For this review, take the finished solid that the model builds, in its own axes (mm). A direction names the side the tool comes from. Coordinates: 2 decimals unless noted, no trailing zeros. Write each loop counter-clockwise with the first axis right and the second up, starting at its lowest first coordinate (ties: lowest second). Pieces come first, ordered by that corner, then holes. Notation, with made-up numbers: M -10,71 L 5,71 A26 cw 5,92 Z; hole C -18,17.5 d3. An arc over 180 degrees is marked long. One line per question, with ' | ' between items.
from build123d import *

# Parameters (mm, degrees)
SKETCH1_W           = 50
SKETCH1_H           = 75
BOSS_EXTRUDE1_DEPTH = 20
SHELL1_T            = -2
FILLET1_R           = 2
SKETCH2_R           = 12.5
BOSS_EXTRUDE2_DEPTH = 1
FILLET2_R           = 2
CUT_EXTRUDE1_DEPTH  = 5
SKETCH4_R           = 2.084715902
SKETCH4_R_2         = 2.544136108
SKETCH4_R_3         = 2.861924979
SKETCH4_R_4         = 2.414925707
BOSS_EXTRUDE3_DEPTH = 7
CHAMFER1_SIZE       = 2
CUT_EXTRUDE2_DEPTH  = 4
SKETCH7_W           = 2
SKETCH7_H           = 1.627577662
BOSS_EXTRUDE4_DEPTH = 3
SKETCH8_W           = 2
SKETCH8_H           = 1.808898565
BOSS_EXTRUDE5_DEPTH = 3
SKETCH9_R           = 0.5
CUT_EXTRUDE3_DEPTH  = 2
CUT_EXTRUDE4_START  = -2
CUT_EXTRUDE4_DEPTH  = 2
SKETCH12_W          = 8.5
SKETCH12_H          = 4
CUT_EXTRUDE5_DEPTH  = 3
SKETCH14_W          = 10
SKETCH14_H          = 2.18902829
CUT_EXTRUDE7_DEPTH  = 3
SKETCH15_W          = 10
SKETCH15_H          = 2.825004844
CUT_EXTRUDE8_DEPTH  = 0.5
CUT_EXTRUDE9_DEPTH  = 3


with BuildPart() as part:
    # Sketch1 → Boss-Extrude1 (new body)
    with BuildSketch(Plane(origin=(0, 0, 0), x_dir=(1, 0, 0), z_dir=(0, 1, 0))):
        with Locations((25, 37.5)):
            Rectangle(SKETCH1_W, SKETCH1_H)
    extrude(amount=BOSS_EXTRUDE1_DEPTH)

    # Shell1
    shell1_openings = [part.faces().sort_by_distance(p)[0] for p in [
        (25, 20, -37.5),
    ]]
    offset(amount=SHELL1_T, openings=shell1_openings, kind=Kind.INTERSECTION)

    # Fillet1
    fillet1_edges = [part.edges().sort_by_distance(p)[0] for p in [
        (0, 10, -75),
        (50, 10, -75),
        (50, 10, 0),
        (0, 10, 0),
    ]]
    fillet(fillet1_edges, radius=FILLET1_R)

    # Sketch2 → Boss-Extrude2 (add)
    with BuildSketch(Plane.XZ):
        with Locations(Location((25, -37.5, 0), (0, 0, 270))):
            Circle(SKETCH2_R)
    extrude(amount=BOSS_EXTRUDE2_DEPTH)

    # Fillet2
    # the kernel refuses this fillet: 2 mm, written as the material it takes off along each edge
    with BuildSketch(Plane(origin=(25, -1, -37.5), x_dir=(0, 0, -1), z_dir=(-1, 0, 0))) as fillet2_piece_1:
        with BuildLine():
            CenterArc((10.767949192, -2), FILLET2_R, 30, 60)
            Line((10.767949192, 0), (10.767949192, 0.04))
            Line((10.767949192, 0.04), (12.5, 0.04))
            Line((12.5, 0.04), (12.54, 0))
            ThreePointArc((12.54, 0), (12.54, -0.5), (12.534641016, -0.98))
            Line((12.534641016, -0.98), (12.5, -1))
        make_face()
    revolve(axis=Axis((25, -1, -37.5), (0, -1, 0)), mode=Mode.SUBTRACT)

    # Sketch3 → Cut-Extrude1 (cut)
    with BuildSketch(Plane.XZ.offset(1)):
        Polygon((33, -40), (33, -37.5), (33, -35), (25.072423756, -35), (25.072423756, -37.5), (25.072423756, -40), align=None)
    extrude(amount=-CUT_EXTRUDE1_DEPTH, mode=Mode.SUBTRACT)

    # Sketch4 → Boss-Extrude3 (add)
    with BuildSketch(Plane(origin=(0, 2, 0), x_dir=(1, 0, 0), z_dir=(0, 1, 0))):
        with Locations(Location((7, 65.5, 0), (0, 0, 90))):
            Circle(SKETCH4_R)
        with Locations(Location((43, 65.5, 0), (0, 0, 90))):
            Circle(SKETCH4_R_2)
        with Locations(Location((43, 9.5, 0), (0, 0, 90))):
            Circle(SKETCH4_R_3)
        with Locations(Location((7, 9.5, 0), (0, 0, 90))):
            Circle(SKETCH4_R_4)
    extrude(amount=BOSS_EXTRUDE3_DEPTH)

    # Chamfer1
    chamfer1_edges = [part.edges().sort_by_distance(p)[0] for p in [
        (33, 2, -37.5),
        (29.036211878, 2, -40),
        (29.036211878, 2, -35),
        (25.072423756, 2, -37.5),
    ]]
    chamfer(chamfer1_edges, length=CHAMFER1_SIZE)

    # Sketch5 → Cut-Extrude2 (cut)
    with BuildSketch(Plane.ZY):
        Polygon((-37.5, 0), (-27.5, 0), (-27.5, 5), (-47.5, 5), (-47.5, 0), align=None)
    cut_extrude2 = extrude(amount=-CUT_EXTRUDE2_DEPTH, mode=Mode.SUBTRACT)

    # Sketch7 → Boss-Extrude4 (add)
    with BuildSketch(Plane(origin=(0, 2, 0), x_dir=(1, 0, 0), z_dir=(0, 1, 0))):
        with Locations((3, 48.313788831)):
            Rectangle(SKETCH7_W, SKETCH7_H)
    boss_extrude4 = extrude(amount=BOSS_EXTRUDE4_DEPTH)

    # Sketch8 → Boss-Extrude5 (add)
    with BuildSketch(Plane(origin=(0, 2, 0), x_dir=(1, 0, 0), z_dir=(0, 1, 0))):
        with Locations((3, 26.595550718)):
            Rectangle(SKETCH8_W, SKETCH8_H)
    boss_extrude5 = extrude(amount=BOSS_EXTRUDE5_DEPTH)

    # Sketch9 → Cut-Extrude3 (cut)
    with BuildSketch(Plane.XY.offset(-47.5)):
        with Locations((2, 4)):
            Circle(SKETCH9_R)
    cut_extrude3 = extrude(amount=-CUT_EXTRUDE3_DEPTH, mode=Mode.SUBTRACT)

    # Sketch10 → Cut-Extrude4 (cut)
    with BuildSketch(Plane(origin=(0, 0, -27.5), x_dir=(-1, 0, 0), z_dir=(0, 0, -1)).offset(CUT_EXTRUDE4_START)):
        with BuildLine():
            ThreePointArc((-1.5, 4), (-1.646446609, 4.353553391), (-2, 4.5))
            Line((-2, 4.5), (-2, 3.5))
            ThreePointArc((-2, 3.5), (-1.646446609, 3.646446609), (-1.5, 4))
        make_face()
        with BuildLine():
            Line((-2, 3.5), (-2, 4.5))
            ThreePointArc((-2, 4.5), (-2.5, 4), (-2, 3.5))
        make_face()
    cut_extrude4 = extrude(amount=CUT_EXTRUDE4_DEPTH, mode=Mode.SUBTRACT)

    # Mirror1: Cut-Extrude2, Boss-Extrude4, Boss-Extrude5, Cut-Extrude3, Cut-Extrude4 across plane
    add(cut_extrude2.mirror(Plane(origin=(25, 0, 0), x_dir=(0, 0, 1), z_dir=(1, 0, 0))), mode=Mode.SUBTRACT)
    add(boss_extrude4.mirror(Plane(origin=(25, 0, 0), x_dir=(0, 0, 1), z_dir=(1, 0, 0))))
    add(boss_extrude5.mirror(Plane(origin=(25, 0, 0), x_dir=(0, 0, 1), z_dir=(1, 0, 0))))
    add(cut_extrude3.mirror(Plane(origin=(25, 0, 0), x_dir=(0, 0, 1), z_dir=(1, 0, 0))), mode=Mode.SUBTRACT)
    add(cut_extrude4.mirror(Plane(origin=(25, 0, 0), x_dir=(0, 0, 1), z_dir=(1, 0, 0))), mode=Mode.SUBTRACT)

    # Sketch12 → Cut-Extrude5 (cut)
    with BuildSketch(Plane.ZY):
        with Locations((-53.834118064, 7.735405472)):
            Rectangle(SKETCH12_W, SKETCH12_H)
    extrude(amount=-CUT_EXTRUDE5_DEPTH, mode=Mode.SUBTRACT)

    # Sketch14 → Cut-Extrude7 (cut)
    with BuildSketch(Plane(origin=(0, 0, -2), x_dir=(-1, 0, 0), z_dir=(0, 0, -1))):
        with Locations((-25, 15.905485855)):
            Rectangle(SKETCH14_W, SKETCH14_H)
    cut_extrude7 = extrude(amount=-CUT_EXTRUDE7_DEPTH, mode=Mode.SUBTRACT)

    # Sketch15 → Cut-Extrude8 (cut)
    with BuildSketch(Plane(origin=(2, 0, 0), x_dir=(0, 0, -1), z_dir=(1, 0, 0))):
        with Locations((37.5, 15.587497578)):
            Rectangle(SKETCH15_W, SKETCH15_H)
    cut_extrude8 = extrude(amount=-CUT_EXTRUDE8_DEPTH, mode=Mode.SUBTRACT)

    # Mirror2: Cut-Extrude7 across plane
    add(cut_extrude7.mirror(Plane.XY.offset(-37.5)), mode=Mode.SUBTRACT)

    # Mirror3: Cut-Extrude8 across plane
    add(cut_extrude8.mirror(Plane(origin=(25, 0, 0), x_dir=(0, 0, 1), z_dir=(1, 0, 0))), mode=Mode.SUBTRACT)

    # Sketch16 → Cut-Extrude9 (cut)
    with BuildSketch(Plane(origin=(0, 0, -75), x_dir=(-1, 0, 0), z_dir=(0, 0, -1))):
        with BuildLine():
            Line((-28.25, 5.769790366), (-21.75, 5.769790366))
            ThreePointArc((-21.75, 5.769790366), (-21.042893219, 5.476897147), (-20.75, 4.769790366))
            Line((-20.75, 4.769790366), (-20.75, 4.269790366))
            ThreePointArc((-20.75, 4.269790366), (-21.042893219, 3.562683585), (-21.75, 3.269790366))
            Line((-21.75, 3.269790366), (-28.25, 3.269790366))
            ThreePointArc((-28.25, 3.269790366), (-28.957106781, 3.562683585), (-29.25, 4.269790366))
            Line((-29.25, 4.269790366), (-29.25, 4.769790366))
            ThreePointArc((-29.25, 4.769790366), (-28.957106781, 5.476897147), (-28.25, 5.769790366))
        make_face()
    extrude(amount=-CUT_EXTRUDE9_DEPTH, mode=Mode.SUBTRACT)


solid = part.part
1) We need section A-A on x = 43. State the section outline as (y, z) points.
Responses:
outline: M 0,-75 L 20,-75 L 20,-73 L 2,-73 L 2,-68.04 L 9,-68.04 L 9,-62.96 L 2,-62.96 L 2,-12.36 L 9,-12.36 L 9,-6.64 L 2,-6.64 L 2,-2 L 20,-2 L 20,0 L 0,0 Z
2) We need section C-C on z = -14. State the section outline as (x, y) points.
Responses:
outline: M 0,0 L 50,0 L 50,20 L 48,20 L 48,2 L 2,2 L 2,20 L 0,20 Z
3) To check wall thickness, follow line 1 along Z through (x, y) = (47.5, 3.75); line 2 along X through (y, z) = (4, -47.95); line 3 along X through (y, z) = (12.25, -59.5). State the ranges of each line that lie inside material, in increasing order. Write a range as [from, to].
Responses:
line 1: [-75, -73], [-49.13, -47.5], [-27.5, -25.69], [-2, 0] | line 2: [0, 1.5], [2.5, 4], [46, 47.5], [48.5, 50] | line 3: [0, 2], [48, 50]
4) The part is to be moulded in two halves that separate along Y. For faces 1 (the flat face through (20, 16, -1)), 2 (the flat face through (1, 8, -49.584)), 3 (the flat face through (20, 2, -38)), 4 (the cylindrical face through (5.24, 5.45, -66.62)), say which applies: +Y half, -Y half, draft (parallel to the pull), parting line (faces both ways), or undercut.
Responses:
face 1: undercut | face 2: undercut | face 3: +Y half | face 4: draft
5) Machinability: for faces 5 (the flat face through (48, 2, -27.5)), 6 (the flat face through (4, 1, -38)), 7 (the flat face through (47, 3, -49.128)), which of the approach directions +Z, -Z, +X, -X, +Y, -Y give a long, thin tool a straight path to every point of the face, cutting with its end or side? Answer none if there is none.
Responses:
face 5: +X, -Y | face 6: -X, +Y, -Y | face 7: +Y
6) We need section B-B on z = -65.5. State the section outline as (x, y) points.
Responses:
outline: M 0,0 L 50,0 L 50,20 L 48,20 L 48,2 L 45.54,2 L 45.54,9 L 40.46,9 L 40.46,2 L 9.08,2 L 9.08,9 L 4.92,9 L 4.92,2 L 2,2 L 2,20 L 0,20 Z
7) Insertion check: pin 1 Ø1 at (x, z) = (49.5, -33) entering from -Y; pin 2 Ø1 at (x, z) = (40.5, -32.5) entering from +Y; pin 3 Ø6 at (x, z) = (42.5, -48) entering from -Y. Each pin has a flat end and moves straight along its axis. Give the tip position at first contact, or say it passes through.
Responses:
pin 1: y = 5 | pin 2: y = 2 | pin 3: y = 0
